The figure shows three views and two pictorial views of one solid part (mm, origin at its lowest corner). Answer the questions. Round coordinates to 2 decimals unless told otherwise and drop trailing zeros. Order: outer loops, then holes, each group sorted by start corner. A loop starts at its lowest first (then second) coordinate and runs counter-clockwise, first axis right, second up. Notation, with made-up numbers: (-6, 19) -> (50, 19) arc R6 ccw to (50, 30) -> close; hole circle Ø9 at (36.25, -25.75). An arc over 180 degrees is marked (long way). Answer in a Markdown table with one row per item. Add a question column.
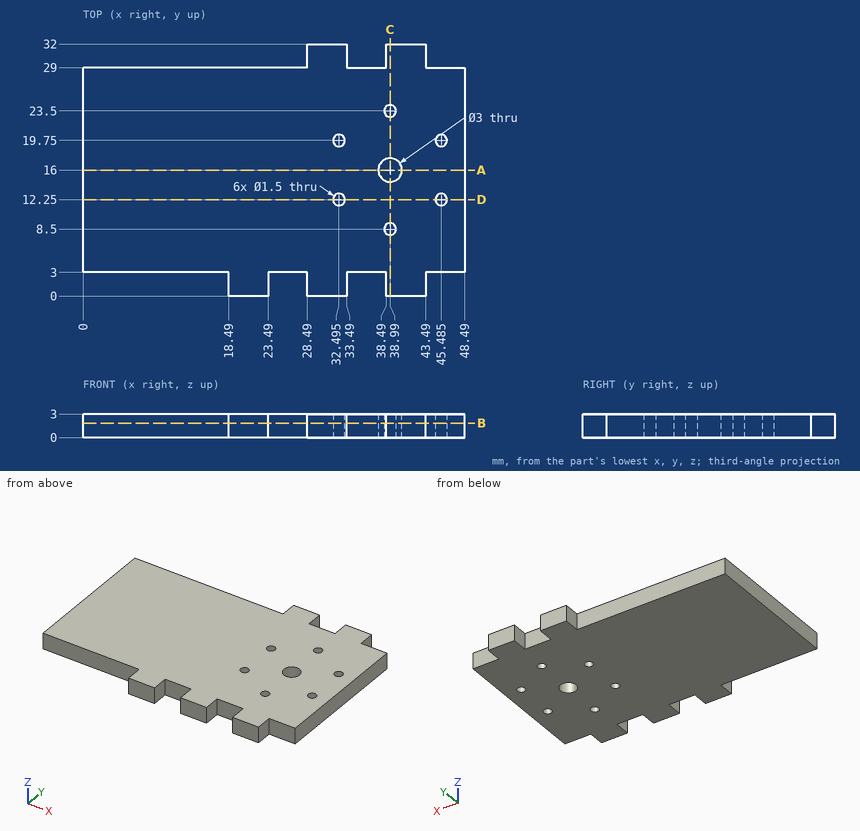
1. The part is cut by section A-A (y = 16). Give the vertices of the cut face in (x, z).
2. The part is cut by section C-C (x = 38.99). Give the vertices of the cut face in (y, z), then the cut area to 3 significant figures.
3. The part is cut by section D-D (y = 12.25). Give the vertices of the cut face in (x, z) (1 decimal).
4. The part is cut by section B-B (z = 1.85). Give the number of separate pieces and of enclosed holes in the cut face, then the cut area to 3 significant figures.
5. Straight lines are drawn through the part: line 1 along Y through (x, z) = (38.99, 0.8); line 2 along X through (y, z) = (2, 0.4); line 3 along Y through (x, z) = (25, 0.9). For each, find the intervals that lie inside material, in ascending order.
6. Each of these flat-tipped pins is pushed along its axis until it touches: pin 1 (1.5 mm diameter, centred on y = 2, z = 1, fed in from -X); pin 2 (1.5 mm diameter, centred on y = 1, z = 2, fed in from +X); pin 3 (1.5 mm diameter, centred on x = 12.5, z = 1.5, fed in from +Y). Where does it stop, or does it pass through?
Report:
| question | item | result |
|---|---|---|
| 1 | outline | (0, 0) -> (37.49, 0) -> (37.49, 3) -> (0, 3) -> close; (40.49, 0) -> (48.49, 0) -> (48.49, 3) -> (40.49, 3) -> close |
| 2 | outline | (0, 0) -> (7.75, 0) -> (7.75, 3) -> (0, 3) -> close; (9.25, 0) -> (14.5, 0) -> (14.5, 3) -> (9.25, 3) -> close; (17.5, 0) -> (22.75, 0) -> (22.75, 3) -> (17.5, 3) -> close; (24.25, 0) -> (32, 0) -> (32, 3) -> (24.25, 3) -> close |
| 2 | area | 78.0 mm^2 |
| 3 | outline | (0, 0) -> (31.7, 0) -> (31.7, 3) -> (0, 3) -> close; (33.2, 0) -> (44.7, 0) -> (44.7, 3) -> (33.2, 3) -> close; (46.2, 0) -> (48.5, 0) -> (48.5, 3) -> (46.2, 3) -> close |
| 4 | separate pieces | 1 |
| 4 | enclosed holes | 7 |
| 4 | area | 1,320 mm^2 |
| 5 | line 1 | y = 0 to 7.75, 9.25 to 14.5, 17.5 to 22.75, 24.25 to 32 |
| 5 | line 2 | x = 18.49 to 23.49, 28.49 to 33.49, 38.49 to 43.49 |
| 5 | line 3 | y = 3 to 29 |
| 6 | pin 1 | stops at x = 18.49 |
| 6 | pin 2 | stops at x = 43.49 |
| 6 | pin 3 | stops at y = 29 |
